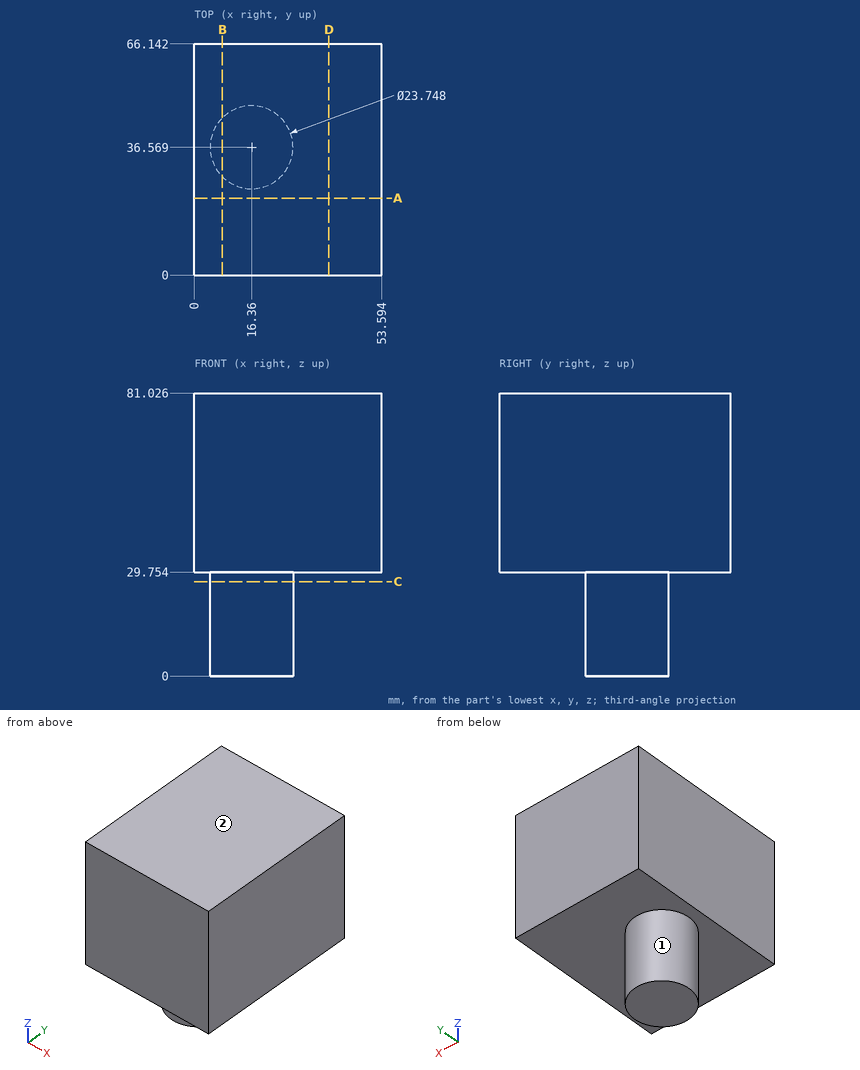
Design review of the part shown in the three views and the two pictorial views. Dimensions are in mm from the part's minimum x, y and z. A direction names the side the tool comes from. Round coordinates to 2 decimals unless told otherwise and drop trailing zeros. Write each loop counter-clockwise with the first axis right and the second up, starting at its lowest first coordinate (ties: lowest second). Pieces come first, ordered by that corner, then holes. Notation, with made-up numbers: (35.25, 60) -> (85.25, 60) arc R18 ccw to (85.25, 87) -> close; hole circle Ø5 at (44.5, 86.25). An arc over 180 degrees is marked (long way). Write item = value, one per line. Start each with the question number.
1) Take a section at D-D, the plane x = 38.5. State the section outline as (y, z) points.
2) Take a section at C-C, the plane z = 27. State the section outline as (x, y) points (1 decimal), plus the area to 3 significant figures.
3) Take a section at A-A, the plane y = 22. State the section outline as (x, z) points, plus the area to 3 significant figures.
4) Clearance check with flat-ended pins moving along their axes: pin 1 (4 mm diameter, centred on y = 38.5, z = 20.5, fed in from +X); pin 2 (3 mm diameter, centred on x = 42.5, y = 48, fed in from -Z); pin 3 (3 mm diameter, centred on x = 17.5, z = 21.5, fed in from +Y). State where each tip first meets the part, or that it passes through.
5) Tool access review of the marked faces 1 and 2: name each direction out of +Z, -Z, +X, -X, +Y, -Y from which nothing blocks a thin tool from reaching the whole face with its end or side.
6) Take a section at B-B, the plane x = 8. State the section outline as (y, z) points.
7) Wall thickness on probe 1 along Z at (x, y) = (34, 42); probe 2 along X at (y, z) = (43, 28.5); probe 3 along X at (y, z) = (46.5, 17.5): over which ranges is each line inside the solid? List them lowest first. Write a range as from..to.
Results list:
q1.outline = (0, 29.75) -> (66.14, 29.75) -> (66.14, 81.03) -> (0, 81.03) -> close
q2.outline = circle Ø23.7 at (16.4, 36.6)
q2.area = 443 mm²
q3.outline = (0, 29.75) -> (53.59, 29.75) -> (53.59, 81.03) -> (0, 81.03) -> close
q3.area = 2,750 mm²
q4.pin_1 = 28.23
q4.pin_2 = 29.75
q4.pin_3 = 48.44
q5.face_1 = -Z
q5.face_2 = +Z, +X, -X, +Y, -Y
q6.outline = (0, 29.75) -> (28.14, 29.75) -> (28.14, 0) -> (45, 0) -> (45, 29.75) -> (66.14, 29.75) -> (66.14, 81.03) -> (0, 81.03) -> close
q7.probe_1 = 29.75..81.03
q7.probe_2 = 6.38..26.34
q7.probe_3 = 9.85..22.87
